from build123d import *

# Parameters (mm, degrees)
F2_T = -2.5
F5_R = 2.5
F8_T = -1
F9_R = 5


with BuildPart() as f1:
    # F0 (on Top) → F1 (revolve)
    with BuildSketch(Plane.XY):
        Polygon((-50, 55), (-30, 0), (0, 0), (0, 55), align=None)
    revolve(axis=Axis((0, 27.5, 0), (0, 1, 0)))

    # F2
    f2_openings = [f1.faces().sort_by_distance(p)[0] for p in [
        (0, 55, 0),
    ]]
    offset(amount=F2_T, openings=f2_openings)

    # F3 (on Top) → F4 (revolve)
    with BuildSketch(Plane.XY):
        Polygon((0, -28.1766057014), (0, 0), (-26.0091759264, 0), (-15.1720196009, -28.1766057014), align=None)
    revolve(axis=Axis((0, -44.4323420525, 0), (0, -1, 0)))

    # F5
    f5_edges = [f1.edges().sort_by_distance(p)[0] for p in [
        (30, 0, 0),
    ]]
    fillet(f5_edges, radius=F5_R)

    # F6 (on Top) → F7 (revolve)
    with BuildSketch(Plane.XY):
        Polygon((0, -28.1766057014), (-10.493944336, -28.1766057014), (-1.9424433219, -145.2080160379), (0, -145.2080160379), align=None)
    revolve(axis=Axis((0, -86.6923108697, 0), (0, -1, 0)))

    # F8
    f8_openings = [f1.faces().sort_by_distance(p)[0] for p in [
        (0, -145.208016, 0),
    ]]
    offset(amount=F8_T, openings=f8_openings, kind=Kind.INTERSECTION)

    # F9
    f9_edges = [f1.edges().sort_by_distance(p)[0] for p in [
        (15.17202, -28.176606, 0),
    ]]
    fillet(f9_edges, radius=F9_R)


solid = f1.part
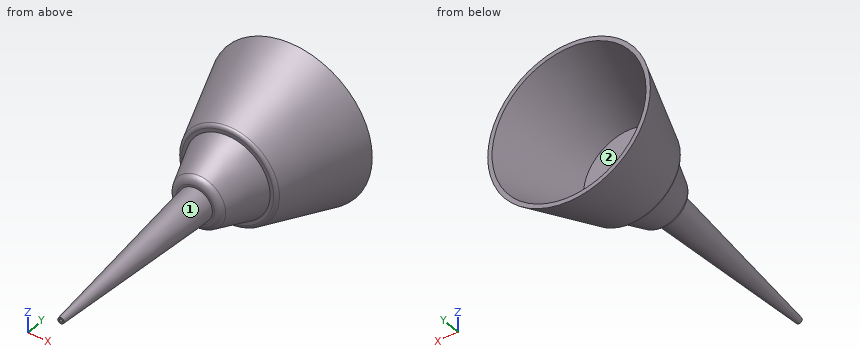
Read the model definition and answer for the solid it produces. Units are mm, in the model's axes. Face numbers are marked on the shaded views. A direction names the side the tool comes from. Round coordinates to 2 decimals unless told otherwise and drop trailing zeros. Order: outer loops, then holes, each group sorted by start corner. A loop starts at its lowest first (then second) coordinate and runs counter-clockwise, first axis right, second up.
1) The part is cut by section A-A on y = -106.5. Write down the section's boundary in (x, z).
2) The part is cut by section B-B on y = -129. Write down the section's boundary in (x, z).
3) Straight lines are drawn through the part: L1, parallel to Y at x = -30.5, z = 24; L2, parallel to X at y = -16, z = 6.5; L3, parallel to X at y = 31.5, z = -34. For each, find the intervals that lie inside material, in ascending order.
4) Flat-ended cylindrical pins translate along their axes: pin 1 (2 mm diameter, centred on x = 2, y = -60.5, fed in from -Z); pin 2 (4 mm diameter, centred on x = 7, z = -4.5, fed in from +Y); pin 3 (4 mm diameter, centred on y = -85.5, z = -2, fed in from +X); pin 4 (11.5 mm diameter, centred on x = 5, z = -1.5, fed in from -Y). Find the tip coordinate at first contact, or state that the pin passes through.
5) For the marked faces 1 and 2, determine the directions among +Z, -Z, +X, -X, +Y, -Y from which every point of the face is accessible in a straight line to the end or side of a thin tool.
Resolved:
1. outline: circle Ø9.54 at (0, 0); hole circle Ø7.54 at (0, 0)
2. outline: circle Ø6.25 at (0, 0); hole circle Ø4.25 at (0, 0)
3. L1: y = 24.23 to 27.15, 28.62 to 31.54
3. L2: x = -18.76 to -17.62, 17.62 to 18.76
3. L3: x = -23.72 to -21.8, -20.8 to -18.68, 18.68 to 20.8, 21.8 to 23.72
4. pin 1: stops at z = -8.09
4. pin 2: stops at y = 2.5
4. pin 3: stops at x = 6.38
4. pin 4: stops at y = -145.21
5. face 1: -Y
5. face 2: +Y
